```python
from build123d import *

# Parameters (mm, degrees)
F2_R     = 6
F3_DEPTH = 40.001
F4_R     = 7
F5_DEPTH = 30
F6_SIZE  = 0.5
F7_SIZE  = 0.99999


# Not quite as in the source:
# - a fillet or chamfer is up to 0.001 mm smaller than in the source, because OpenCascade refuses the exact size


with BuildPart() as f1:
    # F0 (on Top) → F1 (revolve)
    with BuildSketch(Plane.XY):
        Polygon((-50, -40), (0, -40), (0, 0), (-10, 0), (-19.7979589711, -10), (-50, -10), (-50, -15), (-43.7550020016, -20), (-43.7550020016, -30), (-50, -35), align=None)
    revolve(axis=Axis((0, -20, 0), (0, -1, 0)))

    # F2 (on face) → F3 (cut, through all)
    with BuildSketch(Plane(origin=(0, 0, 0), x_dir=(-1, 0, 0), z_dir=(0, 1, 0))):
        Circle(F2_R)
    extrude(amount=-F3_DEPTH, mode=Mode.SUBTRACT)

    # F4 (on face) → F5 (cut)
    with BuildSketch(Plane(origin=(0, -10, 0), x_dir=(-1, 0, 0), z_dir=(0, 1, 0))):
        with Locations((0, 27.7979589711)):
            Circle(F4_R)
        with Locations((26.4374300192, 8.590041731)):
            Circle(F4_R)
        with Locations((16.3392303271, -22.4890212166)):
            Circle(F4_R)
        with Locations((-16.3392303271, -22.4890212166)):
            Circle(F4_R)
        with Locations((-26.4374300192, 8.590041731)):
            Circle(F4_R)
    extrude(amount=-F5_DEPTH, mode=Mode.SUBTRACT)

    # F6
    f6_edges = [f1.edges().sort_by_distance(p)[0] for p in [
        (50, -40, 0),
        (50, -10, 0),
    ]]
    chamfer(f6_edges, length=F6_SIZE)

    # F7 (size 1 in the source; OpenCascade refuses exactly that, so slightly less here)
    f7_edges = [f1.edges().sort_by_distance(p)[0] for p in [
        (7, -10, 27.797959),
        (-19.43743, -10, 8.590042),
        (-9.33923, -10, -22.489021),
        (23.33923, -10, -22.489021),
        (33.43743, -10, 8.590042),
        (-9.33923, -40, -22.489021),
        (-19.43743, -40, 8.590042),
        (33.43743, -40, 8.590042),
        (23.33923, -40, -22.489021),
        (6, -40, 0),
        (7, -40, 27.797959),
    ]]
    chamfer(f7_edges, length=F7_SIZE)


solid = f1.part
```
Here's how the part is built. I have some questions about the finished solid (model axes, mm). A direction names the side the tool comes from. Coordinates: 2 decimals unless noted, no trailing zeros. Order: outer loops, then holes, each group sorted by start corner. A loop starts at its lowest first (then second) coordinate and runs counter-clockwise, first axis right, second up. Notation, with made-up numbers: (59.5, -24.5) - (101.5, -24.5) arc R7 ccw to (101.5, -15.5) - close; hole circle Ø1 at (55.25, -1). An arc over 180 degrees is marked (long way). One line per question, with ' | ' between items. Start each with the question number.
1. Please list where these lines run through material, in increasing order: line 1 along Z through (x, y) = (0, -25.5) (3 decimals); line 2 along Z through (x, y) = (5, -13.5); line 3 along X through (y, z) = (-19.5, -24.5). Write a range as [from, to].
2. Which directions (+Z, -Z, +X, -X, +Y, -Y) give clear straight access to the entire face, cutting with the end or side of a thin tool? Please do faces 1 (the flat face through (21, -10, -1)), 2 (the cylindrical face through (23.21, -24.8, 2.38)), 3 (the conical face through (9.57, -30.313, 43.096)).
3. If we mould it in two halves opening along X, with no side actions, what happens to faces 4 (the cylindrical face through (-47.69, -37.28, -15.02)), 5 (the cylindrical face through (0.91, -24.8, 34.74)), 6 (the flat face through (-10, -40, -1))? For each: released by +X, released by -X, zero draft, split by the parting line, or undercut.
4. If we section it at B-B (y = -21.5): Write out the boundary of the cut face in (x, z) (3 decimals), and give its area (3 significant figures).
5. If we section it at A-A (x = 0): Give the number of separate pieces and of enclosed holes in the cut face, and give its area (3 significant figures).
6. I'm going to push flat-ended pins straight in: pin 1 Ø2 at (x, y) = (1.5, -28.5) entering from +Z; pin 2 Ø3 at (x, y) = (6.5, -20.5) entering from +Z; pin 3 Ø4 at (x, y) = (14, -28.5) entering from +Z. Where does each tip first touch, or does it pass through?
Model answer:
1) line 1: z = [-43.755, -6], [6, 20.798], [34.798, 43.755] | line 2: z = [-49.75, -3.32], [3.32, 22.9], [32.7, 49.75] | line 3: x = [-37, -23.04], [-9.63, 9.63], [23.04, 37]
2) face 1: +Y | face 2: +Y, -Y | face 3: none
3) face 4: split by the parting line | face 5: undercut | face 6: zero draft
4) outline: circle Ø87.51 at (0, 0); hole circle Ø14 at (-26.437, 8.59); hole circle Ø14 at (-16.339, -22.489); hole circle Ø14 at (0, 27.798); hole circle Ø12 at (0, 0); hole circle Ø14 at (16.339, -22.489); hole circle Ø14 at (26.437, 8.59) | area: 5,130 mm²
5) separate pieces: 3 | enclosed holes: 0 | area: 2,210 mm²
6) pin 1: stops at z = 43.75 | pin 2: stops at z = 44.54 | pin 3: stops at z = 42.19
